from build123d import *

# Parameters (mm, degrees)
SKETCH1_W           = 151
SKETCH1_H           = 255
BOSS_EXTRUDE1_DEPTH = 5
SKETCH2_W           = 49.486524855
SKETCH2_H           = 99.222786378
CUT_EXTRUDE1_DEPTH  = 5
SKETCH3_W           = 42
SKETCH3_H           = 67
CUT_EXTRUDE2_DEPTH  = 5
SKETCH4_W           = 120.35
SKETCH4_H           = 95.04721362
CUT_EXTRUDE3_DEPTH  = 5
SKETCH5_W           = 30.1
SKETCH5_H           = 5
SKETCH5_W_2         = 20.1
SKETCH5_H_2         = 5.016666667
CUT_EXTRUDE4_DEPTH  = 5
SKETCH6_R           = 2
CUT_EXTRUDE5_DEPTH  = 10
SKETCH8_R           = 4
SKETCH8_R_2         = 2
BOSS_EXTRUDE2_DEPTH = 5


with BuildPart() as part:
    # Sketch1 → Boss-Extrude1 (new body)
    with BuildSketch(Plane.XY):
        Rectangle(SKETCH1_W, SKETCH1_H)
    extrude(amount=BOSS_EXTRUDE1_DEPTH)

    # Sketch2 → Cut-Extrude1 (cut)
    with BuildSketch(Plane.XY.offset(5)):
        with Locations((-50.756737573, 77.888606811)):
            Rectangle(SKETCH2_W, SKETCH2_H)
    extrude(amount=-CUT_EXTRUDE1_DEPTH, mode=Mode.SUBTRACT)

    # Sketch3 → Cut-Extrude2 (cut)
    with BuildSketch(Plane.XY.offset(5)):
        with Locations((54.5, 94)):
            Rectangle(SKETCH3_W, SKETCH3_H)
    extrude(amount=-CUT_EXTRUDE2_DEPTH, mode=Mode.SUBTRACT)

    # Sketch4 → Cut-Extrude3 (cut)
    with BuildSketch(Plane.XY.offset(5)):
        with Locations((-15.325, -5.976393188)):
            Rectangle(SKETCH4_W, SKETCH4_H)
    extrude(amount=-CUT_EXTRUDE3_DEPTH, mode=Mode.SUBTRACT)

    # Sketch5 → Cut-Extrude4 (cut)
    with BuildSketch(Plane.XY.offset(5)):
        with Locations((40.5, -125)):
            Rectangle(SKETCH5_W, SKETCH5_H)
        with Locations((-40.5, -125)):
            Rectangle(SKETCH5_W, SKETCH5_H)
        with Locations((20.5, -56)):
            Rectangle(SKETCH5_W, SKETCH5_H)
        with Locations((-40.5, -56)):
            Rectangle(SKETCH5_W, SKETCH5_H)
        with Locations((60.5, -7)):
            Rectangle(SKETCH5_W_2, SKETCH5_H)
        with Locations((4.475, 58.004166666)):
            Rectangle(SKETCH5_W, SKETCH5_H_2)
        with Locations((3.5, 125)):
            Rectangle(SKETCH5_W, SKETCH5_H)
    extrude(amount=-CUT_EXTRUDE4_DEPTH, mode=Mode.SUBTRACT)

    # Sketch6 → Cut-Extrude5 (cut)
    with BuildSketch(Plane.XY.offset(5)):
        with Locations((0, -125)):
            Circle(SKETCH6_R)
        with Locations((-2.045010771, -56)):
            Circle(SKETCH6_R)
        with Locations((26.57851787, 58)):
            Circle(SKETCH6_R)
    extrude(amount=-CUT_EXTRUDE5_DEPTH, mode=Mode.SUBTRACT)

    # Sketch8 → Boss-Extrude2 (add)
    with BuildSketch(Plane.XY.offset(5)):
        with Locations((0, -125)):
            Circle(SKETCH8_R)
        with Locations((0, -125)):
            Circle(SKETCH8_R_2, mode=Mode.SUBTRACT)
        with Locations((-2.045010771, -56)):
            Circle(SKETCH8_R)
        with Locations((-2.045010771, -56)):
            Circle(SKETCH8_R_2, mode=Mode.SUBTRACT)
    extrude(amount=-BOSS_EXTRUDE2_DEPTH)


solid = part.part
Geometry check sheet. Reference: the model listing, model coordinates, mm. A direction names the side the tool comes from. Round coordinates to 2 decimals unless told otherwise and drop trailing zeros. Loops run counter-clockwise (first coordinate to the right, second up) from the corner with the lowest first, then second, coordinate; pieces in that order, holes last.
Item 1: Cross-section at C-C on y = 30.5. Record the boundary of the cut face in (x, z).
Item 2: Cross-section at B-B on x = 13. Record the boundary of the cut face in (y, z), then the cut area to 3 significant figures.
Item 3: Mould release check, pull along X, two halves, no side actions. Record for faces 1 (the flat face through (-55.55, -125, 3)), 2 (the flat face through (40, -53.5, 3)), 3 (the flat face through (-75.5, -91, 2)), 4 (the flat face through (-19, 127.5, 2)): pulls with the +X half, pulls with the -X half, needs draft (parallel to the pull), parting line crosses it, or undercut.
Item 4: Gauge pin test, flat ends, axial feed: pin 1 (1.5 mm diameter, centred on y = 125, z = 3, fed in from +X); pin 2 (2.5 mm diameter, centred on y = 98.5, z = 3, fed in from -X); pin 3 (2.5 mm diameter, centred on x = 57, z = 3.5, fed in from +Y). Record the tip position at first contact, or that the pin passes through.
Item 5: Access from +Z, -Z, +X, -X, +Y, -Y to the whole of each face (thin tool, end or side, straight path). Record for faces 5 (the flat face through (-25.45, -125, 3)), 6 (the flat face through (60, -4.5, 3)), 7 (the flat face through (-15, -53.5, 3)), 8 (the flat face through (-14, -127.5, 2)), 9 (the flat face through (33.5, 94, 3)).
Item 6: Cross-section at A-A on x = 66.5. Record the boundary of the cut face in (y, z).
Item 7: Cross-section at D-D on z = 3.65. Count the separate pieces of the cut face and the enclosed holes in it, then the cut area to 3 significant figures.
Item 8: Thickness scan on line 1 (X direction, y = -8.5, z = 0.55); line 2 (Y direction, x = 52, z = 4.65); line 3 (X direction, y = 59, z = 2.3) (3 decimals). Record the ranges inside material, lowest first.
Answer sheet:
1. outline: (44.85, 0) - (75.5, 0) - (75.5, 5) - (44.85, 5) - close
2. outline: (-127.5, 0) - (-58.5, 0) - (-58.5, 5) - (-127.5, 5) - close; (41.55, 0) - (55.5, 0) - (55.5, 5) - (41.55, 5) - close; (60.51, 0) - (122.5, 0) - (122.5, 5) - (60.51, 5) - close
2. area: 725 mm2
3. face 1: undercut
3. face 2: undercut
3. face 3: pulls with the -X half
3. face 4: needs draft
4. pin 1: stops at x = 33.5
4. pin 2: stops at x = -26.01
4. pin 3: stops at y = 60.5
5. face 5: +Z, -Z, -Y
5. face 6: +Z, -Z
5. face 7: +Z, -Z, -X
5. face 8: +Z, -Z, -X, -Y
5. face 9: +Z, -Z, +X, +Y
6. outline: (-127.5, 0) - (-9.5, 0) - (-9.5, 5) - (-127.5, 5) - close; (-4.5, 0) - (60.5, 0) - (60.5, 5) - (-4.5, 5) - close
7. separate pieces: 1
7. enclosed holes: 5
7. area: 19,000 mm2
8. line 1: x = 44.85 to 50.45, 70.55 to 75.5
8. line 2: y = -122.5 to -9.5, -4.5 to 60.5
8. line 3: x = -26.013 to -10.575, 19.525 to 24.846, 28.311 to 75.5
